Read the model definition and answer for the solid it produces. Units are mm, in the model's axes. Coordinates: 2 decimals unless noted, no trailing zeros. Write each loop counter-clockwise with the first axis right and the second up, starting at its lowest first coordinate (ties: lowest second). Pieces come first, ordered by that corner, then holes. Notation, with made-up numbers: (-17, 70.25) -> (-5, 70.25) arc R24 ccw to (-5, 98.25) -> close; hole circle Ø11 at (-25, 77). An arc over 180 degrees is marked (long way). Use CSV: the item, a comma, the result in double quotes. Start each with the question number.
Autodesk Fusion 360 part; units mm, degrees
sketch "Top Panel" plane through (0, 0, 0) normal (0, 0, 1) x (1, 0, 0)
  line L0 (5.15, 228.5) -> (259.15, 228.5)
  line L1 (264.15, 223.5) -> (264.15, 5)
  line L2 (259.15, 0) -> (5.15, 0)
  line L3 (0.15, 5) -> (0.15, 223.5)
  line L4 (10.15, 214) -> (90, 214)
  line L5 (90, 214) -> (90, 19.5)
  line L6 (10.15, 19.5) -> (10.15, 214)
  line L7 (50.075, 27.7654) -> (10.15, 27.7654) construction
  line L8 (50.075, 27.7654) -> (90, 27.7654) construction
  line L9 (50.075, 27.7654) -> (50.075, 12) construction
  arc A0 (36.65, 19.5) -> (63.323, 19.5) centre (49.9865, 27.7752) ccw
  arc A1 (264.15, 223.5) -> (259.15, 228.5) centre (259.15, 223.5) ccw
  arc A2 (259.15, 0) -> (264.15, 5) centre (259.15, 5) ccw
  arc A3 (0.15, 5) -> (5.15, 0) centre (5.15, 5) ccw
  arc A4 (5.15, 228.5) -> (0.15, 223.5) centre (5.15, 223.5) ccw
  circle A5 centre (109.65, 5.1) radius 2.5
  line L10 (109.65, 5.1) -> (107.15, 5.1) construction
  line L11 (109.65, 5.1) -> (109.65, 2.6) construction
  line L12 (109.65, 2.6) -> (109.65, 0) construction
  line L13 (107.15, 5.1) -> (0.15, 5.1) construction
  circle A6 centre (224.65, 5.1) radius 2.5
  line L14 (224.65, 5.1) -> (227.15, 5.1) construction
  line L15 (224.65, 2.6) -> (224.65, 5.1) construction
  line L16 (224.65, 2.6) -> (224.65, 0) construction
  line L17 (227.15, 5.1) -> (264.15, 5.1) construction
  circle A7 centre (109.65, 223.4) radius 2.5
  circle A8 centre (224.65, 223.4) radius 2.5
  line L18 (109.65, 223.4) -> (107.15, 223.4) construction
  line L19 (109.65, 223.4) -> (109.65, 225.9) construction
  line L20 (107.15, 223.4) -> (0.15, 223.4) construction
  line L21 (224.65, 223.4) -> (224.65, 225.9) construction
  line L22 (224.65, 223.4) -> (227.15, 223.4) construction
  line L23 (224.65, 225.9) -> (224.65, 228.5) construction
  line L24 (227.15, 223.4) -> (264.15, 223.4) construction
  line L25 (109.65, 225.9) -> (109.65, 228.5) construction
  line L26 (90, 19.5) -> (63.323, 19.5)
  line L27 (36.65, 19.5) -> (10.15, 19.5)
  point P0 (36.65, 19.5)
  dimension "d1" = 264
  dimension "d2" = 228.5
  dimension "d3" = 79.85
  dimension "d4" = 10
  dimension "d6" = 14.5
  dimension "d8" = 12
  dimension "d9" = 26.5
  dimension "d10" = 5
  dimension "d17" = 2.6
  dimension "d18" = 107
  dimension "d19" = 2.5
  dimension "d20" = 37
extrude "Extrude1" add sketch "Top Panel" along normal blind 3
1) Section B-B, the plane x = 84 is taken. Give the vertices of the cut face in (y, z).
2) Section A-A, the plane y = 117.5 is taken. Give the vertices of the cut face in (x, z), plus the area to 3 significant figures.
3) Section C-C, the plane z = 1 is taken. Give the vertices of the cut face in (x, y).
4) Find the intervals of material crossed by line 1 along Y through (x, z) = (109.65, 2.4); line 2 along X through (y, z) = (223.4, 2.15); line 3 along X through (y, z) = (172, 2.8), in increasing order.
5) The mould has two halves that part along Y. Classify faces 1 (the face through (50.21, 12.08, 1.48)), 2 (the face through (160, 116, 3)): pulls with the +Y half, pulls with the -Y half, needs draft (parallel to the pull), parting line crosses it, or undercut.
The answers:
1,outline,"(0, 0) -> (19.5, 0) -> (19.5, 3) -> (0, 3) -> close; (214, 0) -> (228.5, 0) -> (228.5, 3) -> (214, 3) -> close"
2,outline,"(0.15, 0) -> (10.15, 0) -> (10.15, 3) -> (0.15, 3) -> close; (90, 0) -> (264.15, 0) -> (264.15, 3) -> (90, 3) -> close"
2,area,"552 mm^2"
3,outline,"(0.15, 5) arc R5 ccw to (5.15, 0) -> (259.15, 0) arc R5 ccw to (264.15, 5) -> (264.15, 223.5) arc R5 ccw to (259.15, 228.5) -> (5.15, 228.5) arc R5 ccw to (0.15, 223.5) -> close; hole (10.15, 19.5) -> (36.65, 19.5) arc R15.7 ccw to (63.32, 19.5) -> (90, 19.5) -> (90, 214) -> (10.15, 214) -> close; hole circle Ø5 at (109.65, 5.1); hole circle Ø5 at (109.65, 223.4); hole circle Ø5 at (224.65, 5.1); hole circle Ø5 at (224.65, 223.4)"
4,line 1,"y = 0 to 2.6, 7.6 to 220.9, 225.9 to 228.5"
4,line 2,"x = 0.15 to 107.15, 112.15 to 222.15, 227.15 to 264.15"
4,line 3,"x = 0.15 to 10.15, 90 to 264.15"
5,face 1,"undercut"
5,face 2,"needs draft"
